Autodesk Inventor part; units mm, degrees
ref_plane "Pracovní rovina1" through (0, 0, 6.9) normal (0, 0, 1) x (1, 0, 0)
ref_plane "YZ Plane" through (0, 0, 0) normal (1, 0, 0) x (0, 1, 0)
ref_plane "XZ Plane" through (0, 0, 0) normal (0, 1, 0) x (-1, 0, 0)
sketch "Náčrt1" plane through (0, 0, 0) normal (0, 1, 0) x (-1, 0, 0)
  line L0 (0, -3.7408) -> (0, 22.4445)
  line L1 (9, 0) -> (-1.5, 0)
  line L2 (2.05, 0.3) -> (2.05, 7)
  line L3 (2.05, 7) -> (1.1, 7.5485)
  line L4 (1.1, 7.5485) -> (1.1, 11.6515)
  line L5 (1.1, 11.6515) -> (2.05, 12.2)
  line L6 (2.05, 12.2) -> (2.05, 17.0814)
  arc A0 (3.2, 18.5) -> (2.05, 17.0814) centre (3.5, 17.0814) ccw
  line L7 (3.2, 18.5) -> (3.4, 18.5)
  line L8 (3.4, 18.5) -> (4, 17.9)
  line L9 (4, 17.9) -> (4, 12.65)
  line L10 (4, 12.65) -> (3.375, 12.65)
  line L11 (3.375, 12.65) -> (3.375, 11.4)
  line L12 (3.375, 11.4) -> (5, 11.4)
  line L13 (5, 11.4) -> (5, 6.9)
  line L14 (5, 6.9) -> (3.2, 6.9)
  line L15 (3.2, 6.9) -> (3.2, 5.65)
  line L16 (3.2, 5.65) -> (4, 5.65)
  line L17 (4, 5.65) -> (4, 0.75)
  line L18 (4, 0.75) -> (3.25, 0)
  line L19 (3.25, 0) -> (2.35, 0)
  line L20 (2.05, 0.3) -> (2.35, 0)
  line L21 (5, 11.4) -> (7.5, 10.7301)
  line L22 (7.5, 10.7301) -> (7.5, 11.4)
  line L23 (7.5, 11.4) -> (5, 11.4)
  line L24 (7.5, 6.9) -> (5, 6.9)
  line L25 (7.5, 6.9) -> (5, 6.9)
  line L26 (5, 6.9) -> (5, 7.4)
  line L27 (7.5, 6.9) -> (7.5, 8.1034)
  line L28 (7.5, 8.1034) -> (4.875, 7.4)
  line L29 (4.875, 7.4) -> (4.875, 6.9)
  line L30 (4.875, 6.9) -> (7.5, 6.9)
  line L31 (7.5, 10.7301) -> (7.5, 10.6966)
  line L32 (7.5, 10.6966) -> (4.875, 11.4)
  point P0 (0, 0)
  point P1 (5, 7.4335)
  dimension "d0" = 4.1
  dimension "d1" = 2.2
  dimension "d3" = 60
  dimension "d4" = 60
  dimension "d5" = 0.3
  dimension "d6" = 45
  dimension "d7" = 8
  dimension "d8" = 0.75
  dimension "d9" = 1.45
  dimension "d11" = 1.25
  dimension "d12" = 6.4
  dimension "d13" = 18.5
  dimension "d14" = 6.3
  dimension "d15" = 6.75
  dimension "d16" = 10
  dimension "d17" = 7
  dimension "d18" = 1.25
  dimension "d19" = 7.1
  dimension "d20" = 0.6
  dimension "d21" = 6.4
  dimension "d22" = 4.5
  dimension "d32" = 15
  dimension "d33" = 15
  dimension "d35" = 10
  dimension "d38" = 15
  dimension "d39" = 9.75
  dimension "d40" = 0.5
revolve "Rotace1" add sketch "Náčrt1" angle 360 about axis through (0, 0, -10) along (0, 0, 1) contours L1 L20 L2 L3 L4 L5 L6 A0 L7 L8 L9 L10 L11 L12 L32 L13 L28 L29 L14 L15 L16 L17 L18 | L29 L28 L13 L14 | L32 L12 L13
thread "Závit1"
thread "Závit2"
ref_plane "Pracovní rovina1" through (0, 0, 6.9) normal (0, 0, 1) x (1, 0, 0)
sketch "Náčrt2" plane through (0, 0, 6.9) normal (0, 0, 1) x (1, 0, 0)
  circle A0 centre (0, 0) radius 3.2
  circle A1 centre (0, 0) radius 5
  line L0 (-5.7735, 0) -> (-2.8868, 5)
  line L1 (-2.8868, 5) -> (2.8868, 5)
  line L2 (2.8868, 5) -> (5.7735, 0)
  line L3 (5.7735, 0) -> (2.8868, -5)
  line L4 (2.8868, -5) -> (-2.8868, -5)
  line L5 (-2.8868, -5) -> (-5.7735, 0)
  dimension "d29" = 10
extrude "Vysunutí1" add sketch "Náčrt2" along normal blind 4.5
revolve "Rotace2" cut sketch "Náčrt1" angle 360 about axis through (0, 0, -10) along (0, 0, 1) contours L32 L12 L13 | L13 L21 L31 L32 | L23 L22 L21
revolve "Rotace3" cut sketch "Náčrt1" angle 360 about axis through (0, 0, -10) along (0, 0, 1) contours L29 L28 L13 L14 | L13 L28 L27 L24
equation "\"d30\" = d22"
equation "\"d4\" = d3"
equation "\"d38\" = d33"
equation "\"d28\" = -d19 + d13 - d22"
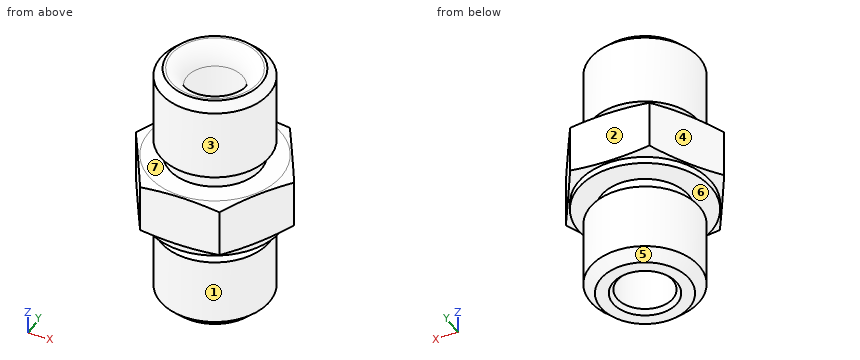
Work out the finished part from the listing and answer in its coordinate system (mm). Face numbers are marked on the shaded views. A direction names the side the tool comes from. Round coordinates to 2 decimals unless told otherwise and drop trailing zeros. Loops run counter-clockwise (first coordinate to the right, second up) from the corner with the lowest first, then second, coordinate; pieces in that order, holes last. Notation, with made-up numbers: M 10.25,-19.75 L 17.25,-19.75 A27 ccw 17.25,18.25 Z; hole C -27,84.5 d6. An arc over 180 degrees is marked long. Use CSV: the item, a comma, the result in double quotes.
Q1. A tool of negligible diameter and unlimited length cuts with its end or side. For the marked faces 1, 2 and 3, from which of +Z, -Z, +X, -X, +Y, -Y can it reach the whole face along a straight path? Write none if from no direction.
Determined:
face 1,"-Z"
face 2,"+Z, -Z, +X, -X, +Y"
face 3,"+Z"
Q2. Section A-A, the plane z = 15.75 is taken. Determine the outline of the cut face in (x, y), then the cut area to 3 significant figures.
Determined:
outline,"C 0,0 d8; hole C 0,0 d4.1"
area,"37.1 mm2"
Q3. Each of these flat-tipped pins is pushed along its axis until it touches: pin 1 (1 mm diameter, centred on y = -1.5, z = 10, fed in from -X); pin 2 (6 mm diameter, centred on x = 1.5, y = -1, fed in from -Z); pin 3 (3 mm diameter, centred on x = 0, y = 0, fed in from -Z); pin 4 (1.5 mm diameter, centred on x = 4.5, y = -2, fed in from +Z). Where does it stop, or does it pass through?
Determined:
pin 1,"x = -5.2"
pin 2,"z = 0"
pin 3,"z = 7.32"
pin 4,"z = 11.4"
Q4. Consider L1, parallel to X at y = 0, z = 1.5; L2, parallel to Z at x = 1.5, y = -3.5; L3, parallel to Z at x = -3.75, y = 0. Determine where each line is inside the solid, lowest interval first.
Determined:
L1,"-4 to -2.05, 2.05 to 4"
L2,"0.56 to 5.65, 6.9 to 11.4, 12.65 to 18.09"
L3,"0.5 to 5.65, 6.9 to 11.4, 12.65 to 18.15"
Q5. The mould has two halves that part along Z. Classify the marked faces 4, 5, 6 and 7: pulls with the +Z half, pulls with the -Z half, needs draft (parallel to the pull), parting line crosses it, or undercut.
Determined:
face 4,"needs draft"
face 5,"pulls with the -Z half"
face 6,"undercut"
face 7,"undercut"
